Check sheet for the modelled part. Datum: model origin and axes. Units: mm. A direction names the side the tool comes from. Give positions to 0.01 mm unless a question says otherwise; leave off trailing zeros. Loops run counter-clockwise (first coordinate to the right, second up) from the corner with the lowest first, then second, coordinate; pieces in that order, holes last. Notation, with made-up numbers: (17.25, 62) -> (60.25, 62) arc R25 ccw to (60.25, 97) -> close; hole circle Ø1 at (49.5, 52). An arc over 180 degrees is marked (long way). Answer as CSV lines item,"result". Start each with the question number.
(1) Gauge pin test, flat ends, axial feed: pin 1 Ø4.5 at (x, z) = (19, 0) entering from +Y; pin 2 Ø5 at (y, z) = (11, -3) entering from -X; pin 3 Ø2 at (x, z) = (-1.5, -3.5) entering from +Y; pin 4 Ø5 at (x, y) = (17.5, 12.5) entering from -Z. Record the tip position at first contact, or that the pin passes through.
(2) Access from +Z, -Z, +X, -X, +Y, -Y to the whole of each face (thin tool, end or side, straight path). Record for faces 4 (the face through (21, 1, 0)), 5 (the face through (-0.66, 5.224, 14.985)).
(3) Section check A-A on z = 0. Enter the section's corners in (x, y), plus the area to 3 significant figures.
(4) Section check D-D on y = 5.75. Enter the section's corners in (x, z).
(5) Material ranges on line 1 (X direction, y = 0.75, z = 0); line 2 (Y direction, x = 12, z = -10); line 3 (Y direction, x = -2, z = 13.5), recorded low to high. Write a range as from..to.
(6) Release check for a two-part mould opening along Z. For faces 1 (the face through (-0.163, 0.592, 16.074)), 2 (the face through (-22.5, 0.6, 0)), 3 (the face through (-17, 1, 0)) record: pulls with the +Z half, pulls with the -Z half, needs draft (parallel to the pull), parting line crosses it, or undercut.
(7) Section check B-B on x = 18.5. Enter the section's corners in (y, z).
from build123d import *

# Parameters (mm, degrees)
SKETCH1_R           = 2
BOSS_EXTRUDE1_DEPTH = 1.2


with BuildPart() as part:
    # Sketch1 → Boss-Extrude1 (new body)
    with BuildSketch(Plane(origin=(0, 0, 0), x_dir=(1, 0, 0), z_dir=(0, 1, 0))):
        with BuildLine():
            ThreePointArc((-10.639111842, -12.050515516), (0, -16.075), (10.639111842, -12.050515516))
            Line((10.639111842, -12.050515516), (21.316447368, -2.623751434))
            ThreePointArc((21.316447368, -2.623751434), (22.5, 0), (21.316447368, 2.623751434))
            Line((21.316447368, 2.623751434), (10.639111842, 12.050515516))
            ThreePointArc((10.639111842, 12.050515516), (0, 16.075), (-10.639111842, 12.050515516))
            Line((-10.639111842, 12.050515516), (-21.316447368, 2.623751434))
            ThreePointArc((-21.316447368, 2.623751434), (-22.5, 0), (-21.316447368, -2.623751434))
            Line((-21.316447368, -2.623751434), (-10.639111842, -12.050515516))
        make_face()
        with Locations(Location((-19, 0, 0), (0, 0, 270))):
            Circle(SKETCH1_R, mode=Mode.SUBTRACT)
        with Locations(Location((19, 0, 0), (0, 0, 270))):
            Circle(SKETCH1_R, mode=Mode.SUBTRACT)
    extrude(amount=BOSS_EXTRUDE1_DEPTH)

    # Sketch3 → Revolve1 (revolve)
    with BuildSketch(Plane.XY, mode=Mode.PRIVATE) as revolve1_sk:
        with BuildLine():
            Line((-15, 1.2), (-15, 9.1375))
            ThreePointArc((-15, 9.1375), (-14.168033936, 12.279760569), (-11.890141265, 14.598634001))
            Line((-11.890141265, 14.598634001), (-7, 17.5))
            ThreePointArc((-7, 17.5), (-4.160829244, 20.777956602), (0, 22))
            Line((0, 22), (0, 1.2))
            Line((0, 1.2), (-15, 1.2))
        make_face()
    revolve(revolve1_sk.sketch.rotate(Axis((0, 1.2, 0), (0, 1, 0)), 270), axis=Axis((0, 1.2, 0), (0, 1, 0)))


solid = part.part
Working result:
1,pin 1,"stops at y = 1.2"
1,pin 2,"stops at x = -14.96"
1,pin 3,"stops at y = 21.47"
1,pin 4,"passes through"
2,face 4,"+Y, -Y"
2,face 5,"+Y"
3,outline,"(-22.5, 0) -> (-21, 0) -> (-21, 1.2) -> (-22.5, 1.2) -> close; (-17, 0) -> (17, 0) -> (17, 1.2) -> (15, 1.2) -> (15, 9.14) arc R6.35 ccw to (11.89, 14.6) -> (7, 17.5) arc R7.69 ccw to (-7, 17.5) -> (-11.89, 14.6) arc R6.35 ccw to (-15, 9.14) -> (-15, 1.2) -> (-17, 1.2) -> close; (21, 0) -> (22.5, 0) -> (22.5, 1.2) -> (21, 1.2) -> close"
3,area,"537 mm^2"
4,outline,"circle Ø30 at (0, 0)"
5,line 1,"x = -22.5..-21, -17..17, 21..22.5"
5,line 2,"y = 0..1.2"
5,line 3,"y = 0..13.06"
6,face 1,"pulls with the +Z half"
6,face 2,"parting line crosses it"
6,face 3,"undercut"
7,outline,"(0, -5.11) -> (1.2, -5.11) -> (1.2, -1.94) -> (0, -1.94) -> close; (0, 1.94) -> (1.2, 1.94) -> (1.2, 5.11) -> (0, 5.11) -> close"
